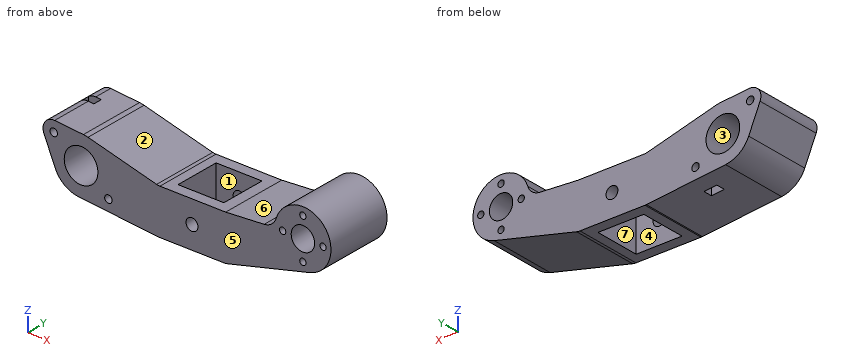
```python
from build123d import *

# Parameters (mm, degrees)
SKETCH1_W           = 30
SKETCH1_H           = 30
SKETCH1_W_2         = 20.4
SKETCH1_H_2         = 20.4
BOSS_EXTRUDE1_DEPTH = 20
SKETCH2_R           = 2.65
CUT_EXTRUDE1_DEPTH  = 40.05124838
SKETCH3_R           = 1.65
SKETCH3_R_2         = 7.5
SKETCH3_R_3         = 1.4
SKETCH3_R_4         = 5.2
BOSS_EXTRUDE2_DEPTH = 30
CUT_EXTRUDE5_START  = -8
CUT_EXTRUDE5_DEPTH  = 4
FILLET1_R           = 6


with BuildPart() as part:
    # Sketch1 → Boss-Extrude1 (new body)
    with BuildSketch(Plane.XY):
        Rectangle(SKETCH1_W, SKETCH1_H)
        Rectangle(SKETCH1_W_2, SKETCH1_H_2, mode=Mode.SUBTRACT)
    extrude(amount=BOSS_EXTRUDE1_DEPTH)

    # Sketch2 → Cut-Extrude1 (cut, through all)
    with BuildSketch(Plane(origin=(0, 15, 0), x_dir=(1, 0, 0), z_dir=(0, 1, 0))):
        with Locations(Location((0, -10, 0), (0, 0, 180))):
            Circle(SKETCH2_R)
    extrude(amount=-CUT_EXTRUDE1_DEPTH, mode=Mode.SUBTRACT)

    # Sketch3 → Boss-Extrude2 (add)
    # profile 1 of 2: a face of its own
    with BuildSketch(Plane(origin=(0, 15, 0), x_dir=(1, 0, 0), z_dir=(0, 1, 0))):
        with BuildLine():
            ThreePointArc((-65.896564393, -22.761029428), (-65.378707028, -27.432622684), (-61.107872478, -29.395256638))
            Line((-61.107872478, -29.395256638), (-48.296614461, -28.315868679))
            ThreePointArc((-48.296614461, -28.315868679), (-47.269565487, -28.186320273), (-46.256757774, -27.972234028))
            Line((-46.256757774, -27.972234028), (-15, -20))
            Line((-15, -20), (-15, 0))
            Line((-15, 0), (-50.542410203, -3.417381881))
            ThreePointArc((-50.542410203, -3.417381881), (-56.721658538, -5.767897005), (-60.8377203, -10.941490233))
            Line((-60.8377203, -10.941490233), (-65.896564393, -22.761029428))
        make_face()
        with Locations(Location((-61.508592346, -24.639111653, 0), (0, 0, 180))):
            Circle(SKETCH3_R, mode=Mode.SUBTRACT)
        with Locations(Location((-49.346059773, -15.86, 0), (0, 0, 180))):
            Circle(SKETCH3_R_2, mode=Mode.SUBTRACT)
        with Locations(Location((-37.1835272, -7.080888347, 0), (0, 0, 180))):
            Circle(SKETCH3_R, mode=Mode.SUBTRACT)
    # profile 2 of 2: a face of its own
    with BuildSketch(Plane(origin=(0, 15, 0), x_dir=(1, 0, 0), z_dir=(0, 1, 0))):
        with BuildLine():
            Line((52.386539741, -9.375418293), (15, 0))
            Line((15, 0), (15, -20))
            Line((15, -20), (36.846059773, -21.5))
            ThreePointArc((36.846059773, -21.5), (57.035142957, -31.355353865), (52.386539741, -9.375418293))
        make_face()
        with Locations(Location((49.346059773, -12.5, 0), (0, 0, 180))):
            Circle(SKETCH3_R_3, mode=Mode.SUBTRACT)
        with Locations(Location((49.346059773, -30.5, 0), (0, 0, 180))):
            Circle(SKETCH3_R_3, mode=Mode.SUBTRACT)
        with Locations(Location((40.346059773, -21.5, 0), (0, 0, 180))):
            Circle(SKETCH3_R_3, mode=Mode.SUBTRACT)
        with Locations(Location((49.346059773, -21.5, 0), (0, 0, 180))):
            Circle(SKETCH3_R_4, mode=Mode.SUBTRACT)
        with Locations(Location((58.346059773, -21.5, 0), (0, 0, 180))):
            Circle(SKETCH3_R_3, mode=Mode.SUBTRACT)
    extrude(amount=-BOSS_EXTRUDE2_DEPTH)

    # Sketch5 → Cut-Extrude5 (cut)
    with BuildSketch(Plane(origin=(0, 15, 0), x_dir=(1, 0, 0), z_dir=(0, 1, 0)).offset(CUT_EXTRUDE5_START)):
        Polygon((-40.041411033, -8.730888347), (-37.1835272, -10.380888347), (-34.325643368, -8.730888347), align=None)
        Polygon((-40.041411033, -8.730888347), (-34.325643368, -8.730888347), (-34.325643368, -5.430888347), (-37.1835272, -3.780888347), (-40.041411033, -5.430888347), align=None)
        Polygon((-37.1835272, -3.780888347), (-34.325643368, -5.430888347), (-34.325643368, 4.153358906), (-40.041411033, 4.153358906), (-40.041411033, -5.430888347), align=None)
        Polygon((-64.366476179, -26.289111653), (-61.508592346, -27.939111653), (-58.650708514, -26.289111653), (-58.650708514, -22.989111653), (-64.366476179, -22.989111653), align=None)
        Polygon((-58.650708514, -26.289111653), (-61.508592346, -27.939111653), (-64.366476179, -26.289111653), (-64.366476179, -31.820729818), (-58.650708514, -31.820729818), align=None)
        Polygon((-64.366476179, -22.989111653), (-58.650708514, -22.989111653), (-61.508592346, -21.339111653), align=None)
    extrude(amount=-CUT_EXTRUDE5_DEPTH, mode=Mode.SUBTRACT)

    # Fillet1
    # the kernel refuses this fillet: 6 mm, written as the material it adds along each edge
    with BuildSketch(Plane(origin=(36.846059773, 15, 21.5), x_dir=(0.15492828046990675, 0, 0.9879257198345622), z_dir=(0, -1, 0))) as fillet1_piece_1:
        with BuildLine():
            CenterArc((4.802776695, 5.927554319), FILLET1_R, 192.840529968, 68.246833251)
            Line((-1.047177652, 4.594124851), (0, 0))
            ThreePointArc((0, 0), (1.936603506, 0.150928502), (3.873207012, 0))
        make_face()
    extrude(amount=30)
    with BuildSketch(Plane(origin=(-15, -15, 20), x_dir=(1, 0, 0), z_dir=(0, 1, 0))) as fillet1_piece_2:
        with BuildLine():
            CenterArc((FILLET1_R * 0.125518959216, -FILLET1_R), FILLET1_R, 90, 14.308582401)
            Line((-FILLET1_R * 0.121625200721, -FILLET1_R * 0.0310212777315), (0, 0))
            Line((0, 0), (FILLET1_R * 0.125518959216, 0))
        make_face()
    extrude(amount=30)
    # the kernel refuses this fillet: 6 mm, written as the material it takes off along each edge
    with BuildSketch(Plane(origin=(15, 16.852100476, 0), x_dir=(-1, 0, 0), z_dir=(0, -1, 0))) as fillet1_2_piece_1:
        with BuildLine():
            CenterArc((FILLET1_R * 0.123473365094, -FILLET1_R), FILLET1_R, 90, 14.07775236)
            Line((-FILLET1_R * 0.119765032297, -FILLET1_R * 0.0300334634457), (0, 0))
            Line((0, 0), (FILLET1_R * 0.123473365094, 0))
        make_face()
    extrude(amount=33.704200953, mode=Mode.SUBTRACT)
    with BuildSketch(Plane(origin=(-15, -15.71946162, 0), x_dir=(1, 0, 0), z_dir=(0, 1, 0))) as fillet1_2_piece_2:
        with BuildLine():
            CenterArc((FILLET1_R * 0.0479641080127, -FILLET1_R), FILLET1_R, 90, 5.492072889)
            Line((-FILLET1_R * 0.0477439263528, -FILLET1_R * 0.004590550498), (0, 0))
            Line((0, 0), (FILLET1_R * 0.0479641080127, 0))
        make_face()
    extrude(amount=31.43892324, mode=Mode.SUBTRACT)


solid = part.part
```
Model file for the job. Use its own axes, mm. Face numbers are marked on the shaded views. A direction names the side the tool comes from. Give positions to 0.01 mm unless a question says otherwise; leave off trailing zeros. Loops run counter-clockwise (first coordinate to the right, second up) from the corner with the lowest first, then second, coordinate; pieces in that order, holes last. Notation, with made-up numbers: (-29, 37.25) -> (-12, 37.25) arc R27 ccw to (-12, 59.25) -> close; hole circle Ø7 at (-38.5, 55). An arc over 180 degrees is marked (long way). Use CSV: the item, a comma, the result in double quotes. Start each with the question number.
1) Tool access for the marked faces 1, 2 and 3: list every direction of +Z, -Z, +X, -X, +Y, -Y with a clear straight run to the whole face (end or side of a thin tool).
2) Mould opens along Y. For the marked faces 4, 5, 6 and 7 say: released by +Y, released by -Y, zero draft, split by the parting line, or undercut.
3) Slice it at C-C on y = -0.5. Give the number of separate pieces and of enclosed holes in the cut face, plus the area to 3 significant figures.
4) Slice it at B-B on z = 30.5. Give the cut face in (x, y).
5) Wall check: line 1 (X direction, y = -7, z = 14); line 2 (X direction, y = -8.75, z = 19.5); line 3 (Y direction, x = 9, z = 7.5). Give the ranges that are in metal, low to high.
6) Slice it at A-A on x = 7. Give the cut face in (y, z), plus the area to 3 significant figures.
7) Flat gauge pins, fed straight in: pin 1 Ø3 at (y, z) = (5, 26.5) entering from +X; pin 2 Ø4 at (x, y) = (20.5, -12) entering from +Z; pin 3 Ø5 at (x, y) = (-26.5, -1) entering from +Z. Where does each tip first touch, or does it go through?
Computed values:
1,face 1,"+Z, -Z"
1,face 2,"+Z, +Y, -Y"
1,face 3,"+Y, -Y"
2,face 4,"undercut"
2,face 5,"released by -Y"
2,face 6,"zero draft"
2,face 7,"undercut"
3,separate pieces,"2"
3,enclosed holes,"8"
3,area,"1,950 mm^2"
4,outline,"(40.67, -15) -> (47.95, -15) -> (47.95, 15) -> (40.67, 15) -> close; (50.75, -15) -> (58.02, -15) -> (58.02, 15) -> (50.75, 15) -> close"
5,line 1,"x = -62.15 to -56.61, -42.08 to -10.2, 10.2 to 59.35"
5,line 2,"x = -64.5 to -55.9, -42.79 to -10.2, 10.2 to 44.55, 54.15 to 61.69"
5,line 3,"y = -15 to -10.2, 10.2 to 15"
6,outline,"(-15, 0) -> (-10.2, 0) -> (-10.2, 20) -> (-15, 20) -> close; (10.2, 0) -> (15, 0) -> (15, 20) -> (10.2, 20) -> close"
6,area,"192 mm^2"
7,pin 1,"stops at x = 61.35"
7,pin 2,"stops at z = 20.51"
7,pin 3,"stops at z = 23.57"
